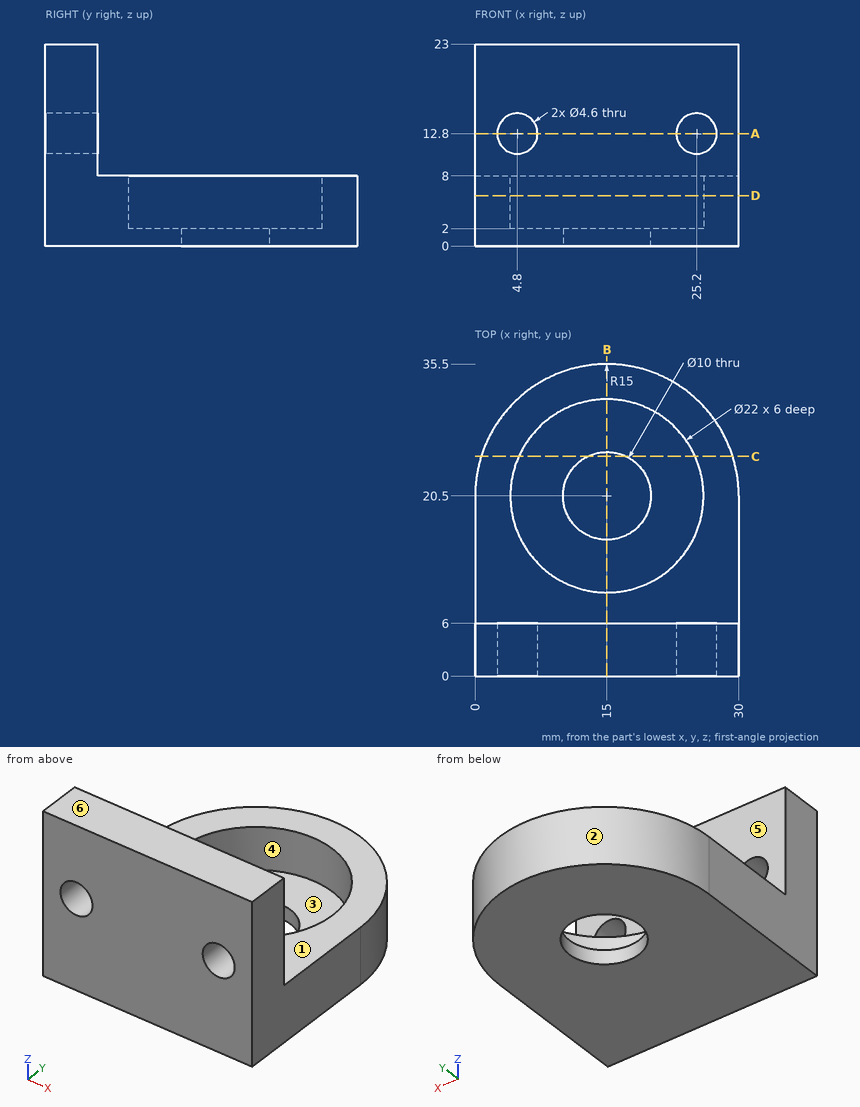
The drawing under review shows one solid part. Ordinate dimensions are in mm from its lowest x, y, z. A direction names the side the tool comes from. Coordinates: 2 decimals unless noted, no trailing zeros. Loops run counter-clockwise (first coordinate to the right, second up) from the corner with the lowest first, then second, coordinate; pieces in that order, holes last.
Item 1: Add section B-B (x = 15). Write out the cut boundary in (y, z).
Completed:
outline: (0, 0) - (15.5, 0) - (15.5, 2) - (9.5, 2) - (9.5, 8) - (6, 8) - (6, 23) - (0, 23) - close; (25.5, 0) - (35.5, 0) - (35.5, 8) - (31.5, 8) - (31.5, 2) - (25.5, 2) - close
Item 2: Clearance check with flat-ended pins moving along their axes: pin 1 (4.5 mm diameter, centred on x = 17.5, z = 16.5, fed in from +Y); pin 2 (13 mm diameter, centred on x = 15, y = 20.5, fed in from +Z); pin 3 (12 mm diameter, centred on x = 4, y = 17.5, fed in from +Z). State where each tip first meets the part, or that it passes through.
Completed:
pin 1: stops at y = 6
pin 2: stops at z = 2
pin 3: stops at z = 8
Item 3: Wall thickness on L1, parallel to Y at x = 15, z = 6; L2, parallel to Y at x = 15, z = 0.55; L3, parallel to Z at x = 4.8, y = 4.65: over which ranges is each line inside the solid? List them lowest first.
Completed:
L1: y = 0 to 9.5, 31.5 to 35.5
L2: y = 0 to 15.5, 25.5 to 35.5
L3: z = 0 to 10.5, 15.1 to 23
Item 4: Draft analysis for pull direction Y (two halves, no side actions). For the marked faces 3, 4, 5 and 6, state which applies: pulls with the +Y half, pulls with the -Y half, needs draft (parallel to the pull), parting line crosses it, or undercut.
Completed:
face 3: undercut
face 4: undercut
face 5: pulls with the +Y half
face 6: needs draft
Item 5: Add section C-C (y = 25). Write out the cut boundary in (x, z).
Completed:
outline: (0.69, 0) - (12.82, 0) - (12.82, 2) - (4.96, 2) - (4.96, 8) - (0.69, 8) - close; (17.18, 0) - (29.31, 0) - (29.31, 8) - (25.04, 8) - (25.04, 2) - (17.18, 2) - close
Item 6: For the marked faces 1 and 2, list the 3-axis set-ups (+Z, -Z, +X, -X, +Y, -Y) from which the entire face can be reached by the end or side of a thin tool; tool diameter is ignored.
Completed:
face 1: +Z, +X, -X, +Y
face 2: +Z, -Z, +Y
Item 7: Add section D-D (z = 5.75). Write out the cut boundary in (x, y).
Completed:
outline: (0, 0) - (30, 0) - (30, 20.5) arc R15 ccw to (0, 20.5) - close; hole circle Ø22 at (15, 20.5)
Item 8: Add section A-A (z = 12.8). Write out the cut boundary in (x, y).
Completed:
outline: (0, 0) - (2.5, 0) - (2.5, 6) - (0, 6) - close; (7.1, 0) - (22.9, 0) - (22.9, 6) - (7.1, 6) - close; (27.5, 0) - (30, 0) - (30, 6) - (27.5, 6) - close
